Geometry check sheet. Reference: the model listing, model coordinates, mm. A direction names the side the tool comes from. Round coordinates to 2 decimals unless told otherwise and drop trailing zeros. Order: outer loops, then holes, each group sorted by start corner. A loop starts at its lowest first (then second) coordinate and runs counter-clockwise, first axis right, second up. Notation, with made-up numbers: (64.5, 60.25) - (81.5, 60.25) arc R17 ccw to (81.5, 77.25) - close; hole circle Ø10 at (-31, 67.5). An arc over 180 degrees is marked (long way). Return JSON: item names as keys, results as strings. Group by question number.
Q1. Sectioned sample at B-B, the plane y = -22. Record the cut outline in (x, z).
Q2. Sectioned sample at D-D, the plane x = -1. Record the cut outline in (y, z).
Q3. Draft check along Y on faces 1 (the flat face through (-25.7, -15.1, 11.9)), 2 (the flat face through (2.4, 6.2, 0)), 3 (the flat face through (25.803, -14.516, 11.917)), 4 (the flat face through (27, -38.1, 6)). Enter one of: pulls with the +Y half, pulls with the -Y half, needs draft (parallel to the pull), parting line crosses it, or undercut.
Q4. Gauge pin test, flat ends, axial feed: pin 1 Ø3 at (y, z) = (-23, 11.5) entering from +X; pin 2 Ø3.5 at (x, z) = (13, 3.5) entering from -Y; pin 3 Ø2 at (y, z) = (3, 8.5) entering from +X. Record the tip position at first contact, or that the pin passes through.
Q5. Sectioned sample at C-C, the plane z = 8.5. Record the cut outline in (x, y) (3 decimals), then the cut area to 3 significant figures.
Q6. Tool access check on faces 5 (the flat face through (-0.417, 6.752, 11.917)), 6 (the flat face through (-30.83, -12.41, 11.92)), 7 (the flat face through (-24.986, -14.545, 5.478)). Record the directions out of +Z, -Z, +X, -X, +Y, -Y that give a thin tool (end or side, any length) a straight path to the whole face; none if there is none.
Q7. Material ranges on line 1 along X through (y, z) = (-29, 6); line 2 along X through (y, z) = (-26, 9.25); line 3 along Y through (x, z) = (8.5, 7.25), recorded low to high.
Q8. Sectioned sample at A-A, the plane x = 24. Record the cut outline in (y, z), then the cut area to 3 significant figures.
```python
from build123d import *

# Parameters (mm, degrees)
F1_DEPTH = 12.7
F2_SIZE  = 1.5875
F3_R     = 3.175


with BuildPart() as f1:
    # F0 (on Top) → F1 (new body)
    with BuildSketch(Plane.XY):
        Polygon((34.29, 12.7), (-34.29, 12.7), (-34.29, 5.94713), (-27.94, 5.94713), (27.94, 5.94713), (34.29, 5.94713), align=None)
        Polygon((-27.94, 5.94713), (-34.29, 5.94713), (-27.94, -38.1), (-21.59, -38.1), align=None)
        Polygon((27.94, -38.1), (34.29, 5.94713), (27.94, 5.94713), (21.59, -38.1), align=None)
    extrude(amount=F1_DEPTH)

    # F2
    f2_edges = [f1.edges().sort_by_distance(p)[0] for p in [
        (-24.765, -16.076435, 12.7),
        (-31.115, -16.076435, 12.7),
        (0, 5.94713, 12.7),
        (24.765, -16.076435, 12.7),
        (31.115, -16.076435, 12.7),
    ]]
    chamfer(f2_edges, length=F2_SIZE)

    # F3
    f3_edges = [f1.edges().sort_by_distance(p)[0] for p in [
        (-21.59, -38.1, 5.55625),
        (21.59, -38.1, 5.55625),
    ]]
    fillet(f3_edges, radius=F3_R)


solid = f1.part
```
Reply:
{
 "1": {"outline": "(-30.26, 0) - (-23.91, 0) - (-23.91, 11.11) - (-25.51, 12.7) - (-28.66, 12.7) - (-30.26, 11.11) - close; (23.91, 0) - (30.26, 0) - (30.26, 11.11) - (28.66, 12.7) - (25.51, 12.7) - (23.91, 11.11) - close"},
 "2": {"outline": "(5.95, 0) - (12.7, 0) - (12.7, 12.7) - (7.53, 12.7) - (5.95, 11.11) - close"},
 "3": {"face 1": "undercut", "face 2": "needs draft", "face 3": "undercut", "face 4": "pulls with the -Y half"},
 "4": {"pin 1": "x = 30.33", "pin 2": "y = 5.95", "pin 3": "x = 34.01"},
 "5": {"outline": "(-34.29, 5.947) - (-27.94, -38.1) - (-25.256, -38.1) arc R3.175 ccw to (-22.113, -34.472) - (-27.94, 5.947) - (27.94, 5.947) - (22.113, -34.472) arc R3.175 ccw to (25.256, -38.1) - (27.94, -38.1) - (34.29, 5.947) - (34.29, 12.7) - (-34.29, 12.7) - close", "area": "1,020 mm^2"},
 "6": {"face 5": "+Z", "face 6": "+Z, -X, -Y", "face 7": "+Z, -Z"},
 "7": {"line 1": "-29.25 to -22.9, 22.9 to 29.25", "line 2": "-29.68 to -23.33, 23.33 to 29.68", "line 3": "5.95 to 12.7"},
 "8": {"outline": "(-37.84, 0) - (-21.38, 0) - (-21.38, 11.11) - (-32.51, 12.7) - (-37.84, 12.7) - close; (5.95, 0) - (12.7, 0) - (12.7, 12.7) - (7.53, 12.7) - (5.95, 11.11) - close", "area": "285 mm^2"}
}
